Geometry: final body of the model. Coordinates: model frame, mm. Give positions to 0.01 mm unless a question says otherwise; leave off trailing zeros. Order: outer loops, then holes, each group sorted by start corner. A loop starts at its lowest first (then second) coordinate and runs counter-clockwise, first axis right, second up. Notation, with made-up numbers: M 5,-29.75 L 53,-29.75 A24 ccw 53,-17.75 Z; hole C 40.25,52.25 d11. An arc over 180 degrees is marked long. Use CSV: the item, a comma, the result in double quotes.
```python
from build123d import *

# Parameters (mm, degrees)
F1_DEPTH = 13.462
F2_W     = 4.9854009032
F2_H     = 1.8919831465


with BuildPart() as f1:
    # F0 (on Top) → F1 (new body)
    with BuildSketch(Plane.XY):
        with BuildLine():
            Line((0, 0), (-32.5159132481, 0))
            Line((-32.5159132481, 0), (-32.5159132481, -7.981837922))
            ThreePointArc((-32.5159132481, -7.981837922), (-16.5119812517, -16.5119812517), (-7.981837922, -32.5159132481))
            Line((-7.981837922, -32.5159132481), (0, -32.5159132481))
            Line((0, -32.5159132481), (0, 0))
        make_face()
    extrude(amount=F1_DEPTH)

    # F3: sweep along a path in F3_path
    with BuildLine(Plane(origin=(-32.5159132481, -7.981837922, 13.462), x_dir=(0, 1, 0), z_dir=(0, 0, 1))) as f3_path:
        ThreePointArc((0, 0), (-8.5301433298, -16.0039319963), (-24.5340753261, -24.5340753261))
    # F2 (on face) → F3 (sweep, cut)
    with BuildSketch(Plane.XZ.offset(32.5159132481)):
        with Locations((-5.4891374703, 6.731)):
            Rectangle(F2_W, F2_H)
    sweep(path=f3_path.line, mode=Mode.SUBTRACT)


solid = f1.part
```
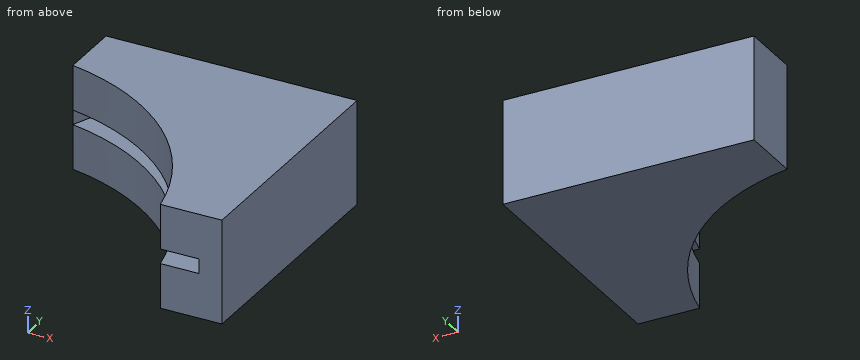
1. Line query: line 1 (Z direction, x = -14.5, y = -14) (3 decimals); line 2 (Y direction, x = -24.5, z = 1.75); line 3 (X direction, y = -16.5, z = 12.25). Output: solid intervals per line, ascending.
Answer:
line 1,"0 to 5.785, 7.677 to 13.462"
line 2,"-10.73 to 0"
line 3,"-16.52 to 0"
2. Section D-D, the plane y = -11.5. Return the cut outline in (x, z) (3 decimals), plus the area to 3 significant figures.
Answer:
outline,"M -23.073,0 L 0,0 L 0,13.462 L -23.073,13.462 L -23.073,7.677 L -14.687,7.677 L -14.687,5.785 L -23.073,5.785 Z"
area,"295 mm2"
3. Section C-C, the plane x = -9. Return the cut outline in (y, z) (3 decimals), plus the area to 3 significant figures.
Answer:
outline,"M -28.66,0 L 0,0 L 0,13.462 L -28.66,13.462 L -28.66,7.677 L -17.865,7.677 L -17.865,5.785 L -28.66,5.785 Z"
area,"365 mm2"
4. Pin query (flat end, axial travel): pin 1 Ø5 at (y, z) = (-27.5, 5.5) entering from -X; pin 2 Ø1.5 at (x, y) = (-23, -14) entering from -Z; pin 3 Ø2 at (x, z) = (-12.5, 2.5) entering from +Y; pin 4 Ø2 at (y, z) = (-17, 3.5) entering from -X. Return the tip coordinate at first contact, or that it passes through.
Answer:
pin 1,"x = -10.49"
pin 2,"through"
pin 3,"y = 0"
pin 4,"x = -17.04"
5. Section B-B, the plane z = 8.5. Return the cut outline in (x, y).
Answer:
outline,"M -32.52,-7.98 A31.12 cw -7.98,-32.52 L 0,-32.52 L 0,0 L -32.52,0 Z"
6. Section A-A, the plane y = -4.5. Return the cut outline in (x, z) (3 decimals), plus the area to 3 significant figures.
Answer:
outline,"M -32.516,0 L 0,0 L 0,13.462 L -32.516,13.462 Z; hole M -31.093,5.785 L -26.66,5.785 L -26.66,7.677 L -31.093,7.677 Z"
area,"429 mm2"
